from build123d import *

# Parameters (mm, degrees)
F0_W      = 25.4
F0_H      = 25.4
F1_DEPTH  = 19.05
F2_W      = 33.1137652975
F2_H      = 28.659734875
F3_DEPTH  = 19.051
F5_DEPTH  = 12.7
F7_DEPTH  = 2.54
F9_DEPTH  = 12.7
F12_DEPTH = 25.4
F15_DEPTH = 25.4
F17_DEPTH = 5.08
F18_R     = 1.27
F20_R     = 1.5875
F21_DEPTH = 12.7
F22_R     = 0.254


with BuildPart() as f1:
    # F0 (on Top) → F1 (new body)
    with BuildSketch(Plane.XY):
        Rectangle(F0_W, F0_H)
    extrude(amount=F1_DEPTH)

    # F2 (on face) → F3 (cut, through all)
    with BuildSketch(Plane.XY.offset(19.05)):
        with Locations((-1.1700320756, 0)):
            Rectangle(F2_W, F2_H)
        with BuildLine():
            ThreePointArc((-12.065, 10.0208269432), (0, 11.8638118431), (12.065, 10.0208269432))
            Line((12.065, 10.0208269432), (12.3786535114, 6.750300061))
            Line((12.3786535114, 6.750300061), (12.7, 6.5362956375))
            Line((12.7, 6.5362956375), (12.7, 1.6182865947))
            Line((12.7, 1.6182865947), (12.3786535114, 1.0663146386))
            Line((12.3786535114, 1.0663146386), (12.7, -8.5426112637))
            Line((12.7, -8.5426112637), (4.8173773102, -12.7))
            Line((4.8173773102, -12.7), (0, -12.7))
            Line((0, -12.7), (-4.8173773102, -12.7))
            Line((-4.8173773102, -12.7), (-12.7, -8.5426112637))
            Line((-12.7, -8.5426112637), (-12.3786535114, 1.0663146386))
            Line((-12.3786535114, 1.0663146386), (-12.7, 1.6182865947))
            Line((-12.7, 1.6182865947), (-12.7, 6.5362956375))
            Line((-12.7, 6.5362956375), (-12.3786535114, 6.750300061))
            Line((-12.3786535114, 6.750300061), (-12.065, 10.0208269432))
        make_face(mode=Mode.SUBTRACT)
    extrude(amount=-F3_DEPTH, mode=Mode.SUBTRACT)

    # F4 (on Right) → F5 (cut, symmetric)
    with BuildSketch(Plane.YZ):
        Polygon((13.4258409962, 23.2345554978), (6.619815249, 19.5569172502), (12.7253746614, 12.7713512629), align=None)
    extrude(amount=F5_DEPTH, both=True, mode=Mode.SUBTRACT)

    # F6 (on face) → F7 (cut)
    with BuildSketch(Plane.XY.offset(19.05)):
        with BuildLine():
            ThreePointArc((11.0015488178, 6.9544261182), (0, 6.3570296668), (-11.0015488178, 6.9544261182))
            Line((-11.0015488178, 6.9544261182), (-11.1053383224, 6.0839187998))
            Line((-11.1053383224, 6.0839187998), (-11.5596242249, 2.2737146355))
            add(Edge.make_bspline(
                [(-2.4099256195, 1.3795604811), (-7.9047118703, 0.0093029614), (-9.4140619773, 0.61575824), (-11.5596242249, 2.2737146355)],
                knots=[0, 0, 0, 0, 0.380461969, 0.380461969, 0.380461969, 0.380461969], degree=3))
            Line((-2.4099256195, 1.3795604811), (-1.8782533274, 2.4663225251))
            Line((-1.8782533274, 2.4663225251), (0, 2.3830392409))
            Line((0, 2.3830392409), (1.8782533274, 2.4663225251))
            Line((1.8782533274, 2.4663225251), (2.4099256195, 1.3795604811))
            add(Edge.make_bspline(
                [(2.4099256195, 1.3795604811), (7.9047118703, 0.0093029614), (9.4140619773, 0.61575824), (11.5596242249, 2.2737146355)],
                knots=[0, 0, 0, 0, 0.380461969, 0.380461969, 0.380461969, 0.380461969], degree=3))
            Line((11.5596242249, 2.2737146355), (11.1053383224, 6.0839187998))
            Line((11.1053383224, 6.0839187998), (11.0015488178, 6.9544261182))
        make_face()
    extrude(amount=-F7_DEPTH, mode=Mode.SUBTRACT)

    # F8 (on Right) → F9 (cut, symmetric)
    with BuildSketch(Plane.YZ):
        Polygon((16.2616688758, -2.9984780122), (12.367782183, 5.9512541629), (7.8229103237, -1.7573904479), align=None)
        Polygon((-14.0263205394, -2.3636263795), (-5.847228691, -0.8765184903), (-8.5426112637, 6.5125478432), (-13.6080719531, 6.5125478432), align=None)
    extrude(amount=F9_DEPTH, both=True, mode=Mode.SUBTRACT)

    # F11 (on 3pt) → F12 (cut)
    with BuildSketch(Plane(origin=(13.5235138631, -7.4279156196, 6.0395065555), x_dir=(-0.409334057, -0.8938834922, -0.1828057224), z_dir=(-0.8161889166, 0.4482993446, -0.3645042525))):
        Polygon((9.3890596181, -6.6504105926), (10.8706550673, 19.4640029222), (-6.7497892305, 22.2047120333), (-12.2956875712, 3.634221619), (-6.1068134382, -4.8245443031), align=None)
    extrude(amount=-F12_DEPTH, mode=Mode.SUBTRACT)

    # F14 (on 3pt) → F15 (cut)
    with BuildSketch(Plane(origin=(-13.5235138631, -7.4279156196, 6.0395065555), x_dir=(0.409334057, -0.8938834922, -0.1828057224), z_dir=(-0.8161889166, -0.4482993446, 0.3645042525))):
        Polygon((12.0957437903, 22.2065132111), (-11.2094106153, 21.0766065866), (-8.9160036296, -5.990778096), (12.0957437903, -5.990778096), align=None)
    extrude(amount=F15_DEPTH, mode=Mode.SUBTRACT)

    # F16 (on face) → F17 (cut)
    with BuildSketch(Plane.XY.offset(19.05)):
        with BuildLine():
            Line((5.2999914624, -5.4918094538), (0, -5.4918094538))
            Line((0, -5.4918094538), (-5.2999914624, -5.4918094538))
            Line((-5.2999914624, -5.4918094538), (-6.5067803222, -6.403681509))
            ThreePointArc((-6.5067803222, -6.403681509), (-6.2496472485, -8.0992009526), (-4.9241394059, -9.1872876037))
            Line((-4.9241394059, -9.1872876037), (-4.2353287011, -8.6668094538))
            Line((-4.2353287011, -8.6668094538), (0, -8.6668094538))
            Line((0, -8.6668094538), (4.2353287011, -8.6668094538))
            Line((4.2353287011, -8.6668094538), (4.9241394059, -9.1872876037))
            ThreePointArc((4.9241394059, -9.1872876037), (6.2496472485, -8.0992009526), (6.5067803222, -6.403681509))
            Line((6.5067803222, -6.403681509), (5.2999914624, -5.4918094538))
        make_face()
    extrude(amount=-F17_DEPTH, mode=Mode.SUBTRACT)

    # F18
    f18_edges = [f1.edges().sort_by_distance(p)[0] for p in [
        (-11.001549, 6.954426, 17.78),
        (11.001549, 6.954426, 17.78),
        (11.559624, 2.273715, 17.78),
        (-11.559624, 2.273715, 17.78),
    ]]
    fillet(f18_edges, radius=F18_R)

    # F20 (on face) → F21 (cut, symmetric)
    with BuildSketch(Plane(origin=(-4.0520275589, -3.3428374331, 0), x_dir=(-0.6363732922, 0.7713812501, 0), z_dir=(0.7713812501, 0.6363732922, 0))):
        with Locations((12.3976198956, 8.7611014023)):
            Circle(F20_R)
    extrude(amount=F21_DEPTH, both=True, mode=Mode.SUBTRACT)

    # F22
    f22_edges = [f1.edges().sort_by_distance(p)[0] for p in [
        (-4.235329, -8.666809, 16.51),
        (-4.924139, -9.187288, 16.51),
        (-6.50678, -6.403682, 16.51),
        (-5.299991, -5.491809, 16.51),
        (4.235329, -8.666809, 16.51),
        (4.924139, -9.187288, 16.51),
        (6.50678, -6.403682, 16.51),
        (5.299991, -5.491809, 16.51),
    ]]
    fillet(f22_edges, radius=F22_R)


solid = f1.part
Here's how the part is built. I have some questions about the finished solid (model axes, mm). A direction names the side the tool comes from. Give positions to 0.01 mm unless a question says otherwise; leave off trailing zeros. Order: outer loops, then holes, each group sorted by start corner. A loop starts at its lowest first (then second) coordinate and runs counter-clockwise, first axis right, second up. Notation, with made-up numbers: (2.25, -13) -> (27.25, -13) arc R21 cw to (27.25, 11) -> close; hole circle Ø1 at (16, -31). An arc over 180 degrees is marked (long way). Use a Markdown table: item, result. Add a question column.
Item 1: I need wall thicknesses on line 1 (Y direction, x = 3.75, z = 18); line 2 (Y direction, x = -1.25, z = 14.75); line 3 (Z direction, x = 8.5, y = 5.25). Which ranges of each line are inside material? Lowest first, please.
Item 2: If we mould it in two halves opening along Y, with no side actions, what happens to faces 1 (the face through (0.926, 2.424, 17.798)), 2 (the face through (7.062, -11.516, 10.083)), 3 (the face through (-12.7, 3, 9))? For each: pulls with the +Y half, pulls with the -Y half, needs draft (parallel to the pull), parting line crosses it, or undercut.
Item 3: For faces 4 (the face through (-11.31, 4.38, 17.8)), 5 (the face through (0, -10, 6.513)), 6 (the face through (0, -3, 19.05)), which set-ups out of +Z, -Z, +X, -X, +Y, -Y let a thin tool reach every point of the face, with its end or its side?
Item 4: Will these pins go through, and if not, where does the flat tip stop? pin 1 (1.5 mm diameter, centred on x = -2, z = 16, fed in from +Y); pin 2 (5 mm diameter, centred on y = -10, z = 10.5, fed in from +X); pin 3 (1 mm diameter, centred on y = -10, z = 12.5, fed in from +X).
Item 5: Imagine slicing it at C-C on y = -2. Please give me the cut outline in (x, z).
Item 6: Imagine slicing it at A-A on z = 7.75. Please give me the cut outline in (x, y) (3 decimals).
Item 7: Imagine slicing it at D-D on x = -0.75. Please give me the cut outline in (y, z).
Data:
| question | item | result |
|---|---|---|
| 1 | line 1 | y = -12.7 to -8.67, -5.49 to 1.07, 6.43 to 8.02 |
| 1 | line 2 | y = -12.7 to -8.67, -5.49 to 10.95 |
| 1 | line 3 | z = 0 to 16.51 |
| 2 | face 1 | undercut |
| 2 | face 2 | pulls with the -Y half |
| 2 | face 3 | needs draft |
| 3 | face 4 | +Z |
| 3 | face 5 | -Z, +X, -X, -Y |
| 3 | face 6 | +Z, +X, -X, +Y, -Y |
| 4 | pin 1 | stops at y = 10.5 |
| 4 | pin 2 | stops at x = 11.89 |
| 4 | pin 3 | stops at x = 9.58 |
| 5 | outline | (-12.48, 0) -> (12.48, 0) -> (12.48, 15.05) -> (10.69, 19.05) -> (-10.69, 19.05) -> (-12.48, 15.05) -> close |
| 6 | outline | (-12.7, 1.618) -> (-12.379, 1.066) -> (-12.668, -7.594) -> (-11.922, -8.953) -> (-4.817, -12.7) -> (4.817, -12.7) -> (11.922, -8.953) -> (12.668, -7.594) -> (12.379, 1.066) -> (12.7, 1.618) -> (12.7, 6.536) -> (12.379, 6.75) -> (12.065, 10.021) arc R40.413 ccw to (-3.346, 11.725) -> (-12.7, 4.008) -> close; (-12.306, 7.506) -> (-7.991, 11.066) arc R40.413 ccw to (-12.065, 10.021) -> close |
| 7 | outline | (-12.7, 6.51) -> (-8.54, 6.51) -> (-6.17, 0) -> (8.86, 0) -> (11.86, 5.08) -> (11.86, 13.74) -> (7.08, 19.05) -> (6.36, 19.05) -> (6.36, 16.51) -> (2.42, 16.51) -> (2.42, 19.05) -> (-5.49, 19.05) -> (-5.49, 13.97) -> (-8.67, 13.97) -> (-8.67, 19.05) -> (-12.7, 19.05) -> close |
